Check sheet for the modelled part. Datum: model origin and axes. Units: mm. A direction names the side the tool comes from. Round coordinates to 2 decimals unless told otherwise and drop trailing zeros. Order: outer loops, then holes, each group sorted by start corner. A loop starts at its lowest first (then second) coordinate and runs counter-clockwise, first axis right, second up.
Q1. Cross-section at B-B on y = 11. Record the cut outline in (x, z).
Q2. Cross-section at C-C on z = 15. Record the cut outline in (x, y), then the cut area to 3 significant figures.
Q3. Scan lines: probe 1 along Z at (x, y) = (-15.5, 15.5); probe 2 along Y at (x, z) = (-22.5, 5.5); probe 3 along X at (y, z) = (10, 6.5). Record each from-to range of solid material in increasing order.
Q4. Cross-section at D-D on y = 0. Record the cut outline in (x, z), then the cut area to 3 significant figures.
Q5. Depth check by flat-ended pin: P1, Ø14.5, axis at x = -16.25, y = 9.28, coming from the -Z side. Enter the tip coordinate at first touch or a pass-through.
Q6. Cross-section at A-A on x = -15. Record the cut outline in (y, z).
Q7. Set-up check for faces 4 (the flat face through (-17, -2.718, 9)), 5 (the cylindrical face through (-18.635, -1.456, 4.93)): record each of +Z, -Z, +X, -X, +Y, -Y from which the full face is reachable in a straight line by a thin tool's end or side.
Q8. Mould release check, pull along Y, two halves, no side actions. Record for faces 1 (the cylindrical face through (-64.824, -1.214, 9.126)), 2 (the cylindrical face through (-12.093, 7.559, 13.944)), 3 (the flat face through (-17, 23, 0)): +Y half, -Y half, draft (parallel to the pull), parting line (faces both ways), or undercut.
from build123d import *

# Parameters (mm, degrees)
F0_W     = 100
F0_H     = 35
F0_R     = 11
F0_R_2   = 4.5
F1_DEPTH = 18
F2_DEPTH = 10
F3_R     = 5


with BuildPart() as f1:
    # F0 (on Top) → F1 (new body)
    with BuildSketch(Plane.XY):
        with Locations((-16.250001, 14.782052)):
            Rectangle(F0_W, F0_H)
        with Locations((-16.250001, 9.282052)):
            Circle(F0_R, mode=Mode.SUBTRACT)
        with Locations((-16.250001, 9.282052)):
            Circle(F0_R)
        with Locations((-16.250001, 9.282052)):
            Circle(F0_R_2, mode=Mode.SUBTRACT)
    extrude(amount=F1_DEPTH)

    # F0 (on Top) → F2 (cut)
    with BuildSketch(Plane.XY):
        with Locations((-16.250001, 9.282052)):
            Circle(F0_R)
        with Locations((-16.250001, 9.282052)):
            Circle(F0_R_2, mode=Mode.SUBTRACT)
    extrude(amount=F2_DEPTH, mode=Mode.SUBTRACT)

    # F3
    f3_edges = [f1.edges().sort_by_distance(p)[0] for p in [
        (33.749999, -2.717948, 9),
        (-66.250001, -2.717948, 9),
    ]]
    fillet(f3_edges, radius=F3_R)


solid = f1.part
Results found:
1. outline: (-66.25, 0) - (-27.12, 0) - (-27.12, 10) - (-20.41, 10) - (-20.41, 18) - (-66.25, 18) - close; (-12.09, 10) - (-5.38, 10) - (-5.38, 0) - (33.75, 0) - (33.75, 18) - (-12.09, 18) - close
2. outline: (-66.25, 2.28) arc R5 ccw to (-61.25, -2.72) - (28.75, -2.72) arc R5 ccw to (33.75, 2.28) - (33.75, 32.28) - (-66.25, 32.28) - close; hole circle Ø9 at (-16.25, 9.28)
2. area: 3,430 mm2
3. probe 1: z = 10 to 18
3. probe 2: y = -2.72 to 0.23, 18.33 to 32.28
3. probe 3: x = -66.25 to -27.23, -5.27 to 33.75
4. outline: (-65.7, 0) - (-22.15, 0) - (-22.15, 10) - (-10.35, 10) - (-10.35, 0) - (33.2, 0) - (33.2, 18) - (-65.7, 18) - close
4. area: 1,660 mm2
5. P1: stops at z = 10
6. outline: (-2.72, 0) - (-1.65, 0) - (-1.65, 10) - (4.96, 10) - (4.96, 18) - (-2.72, 18) - close; (13.6, 10) - (20.21, 10) - (20.21, 0) - (32.28, 0) - (32.28, 18) - (13.6, 18) - close
7. face 4: +Z, -Z, +X, -X, -Y
7. face 5: -Z
8. face 1: -Y half
8. face 2: undercut
8. face 3: draft
